For this review, use the dimensioned drawing (mm, ordinates from the lowest corner) and the shaded views. Give positions to 0.01 mm unless a question says otherwise; leave off trailing zeros. Write each loop counter-clockwise with the first axis right and the second up, starting at its lowest first coordinate (ties: lowest second). Pieces come first, ordered by that corner, then holes. Notation, with made-up numbers: (30, -6.5) - (74, -6.5) arc R28 ccw to (74, 27.5) - close; hole circle Ø4 at (31.25, 75.5). An arc over 180 degrees is marked (long way). Use a Markdown table: item, result. Add a question column.
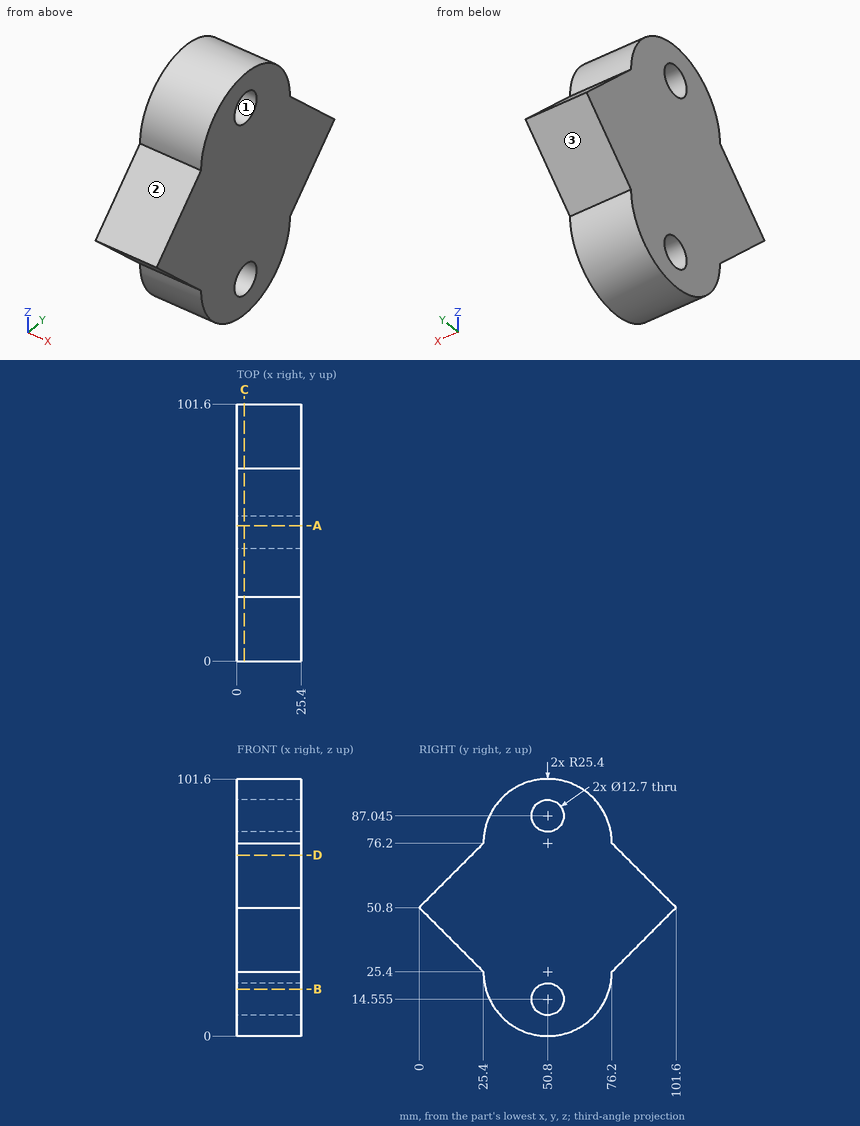
(1) Insertion check: pin 1 (5 mm diameter, centred on x = 10.5, y = 90, fed in from +Z); pin 2 (2 mm diameter, centred on x = 12, y = 45, fed in from +Z); pin 3 (10 mm diameter, centred on y = 26, z = 67, fed in from -X); pin 4 (1.5 mm diameter, centred on y = 54, z = 82.5, fed in from +X). Each pin has a flat end and moves straight along its axis. Give the tip position at first contact, or say it passes through.
(2) Add section C-C (x = 3). State the section outline as (y, z) points (3 decimals).
(3) For line 1 along Z through (x, y) = (16.5, 50.8) (3 decimals); line 2 along Z through (x, y) = (17.5, 45); line 3 along Y through (x, z) = (8.75, 77), list the stretches that pass through material, from the lowest coordinate up.
(4) Add section B-B (z = 18.5). State the section outline as (x, y) points (3 decimals), and give its area (3 significant figures).
(5) Add section A-A (y = 53.5). State the section outline as (x, z) points.
(6) Add section D-D (z = 71.5). State the section outline as (x, y) points.
(7) Mouldability with a two-part tool opening along Z and no side actions: class the marked faces 1, 2 and 3 as +Z half, -Z half, draft (parallel to the pull), parting line (faces both ways), or undercut.
Answers follow:
| question | item | result |
|---|---|---|
| 1 | pin 1 | z = 64.9 |
| 1 | pin 2 | z = 101.14 |
| 1 | pin 3 | x = 0 |
| 1 | pin 4 | through |
| 2 | outline | (0, 50.8) - (25.4, 25.4) arc R25.4 ccw to (76.2, 25.4) - (101.6, 50.8) - (76.2, 76.2) arc R25.4 ccw to (25.4, 76.2) - close; hole circle Ø12.7 at (50.8, 14.555); hole circle Ø12.7 at (50.8, 87.045) |
| 3 | line 1 | 0 to 8.205, 20.905 to 80.695, 93.395 to 101.6 |
| 3 | line 2 | 0.67 to 11.97, 17.14 to 84.46, 89.63 to 100.93 |
| 3 | line 3 | 25.41 to 76.19 |
| 4 | outline | (0, 26.355) - (25.4, 26.355) - (25.4, 45.824) - (0, 45.824) - close; (0, 55.776) - (25.4, 55.776) - (25.4, 75.245) - (0, 75.245) - close |
| 4 | area | 989 mm^2 |
| 5 | outline | (0, 0.14) - (25.4, 0.14) - (25.4, 8.81) - (0, 8.81) - close; (0, 20.3) - (25.4, 20.3) - (25.4, 81.3) - (0, 81.3) - close; (0, 92.79) - (25.4, 92.79) - (25.4, 101.46) - (0, 101.46) - close |
| 6 | outline | (0, 20.7) - (25.4, 20.7) - (25.4, 80.9) - (0, 80.9) - close |
| 7 | face 1 | undercut |
| 7 | face 2 | +Z half |
| 7 | face 3 | -Z half |
